Part model, mm, in its own coordinate system. Face numbers are marked on the shaded views. A direction names the side the tool comes from. Coordinates: 2 decimals unless noted, no trailing zeros. Loops run counter-clockwise (first coordinate to the right, second up) from the corner with the lowest first, then second, coordinate; pieces in that order, holes last. Notation, with made-up numbers: (68, 80.5) - (125, 80.5) arc R30 cw to (125, 102.5) - close; hole circle Ø9 at (-23.5, 59.25). An arc over 180 degrees is marked (long way). Use a Markdown table: item, result. Add a question column.
1) Pull direction X, two halves, no side cores. Call the marked faces 3, 4 and 5: +X half, -X half, draft (parallel to the pull), parting line (faces both ways), or undercut.
2) Drop flat-ended pins along their axis: P1, Ø1.5, axis at x = 131, y = 53.5, coming from the +Z side; P2, Ø1.5, axis at x = 109, z = -30, coming from the +Y side. Give the stop position or say it passes through.
3) Probe probe 1 along X at (y, z) = (14.5, -99); probe 2 along Y at (x, z) = (57, -85.5); probe 3 along Z at (x, y) = (65, 60.5). List the from-to ranges inside material, lowest first. Write a range as [from, to].
4) Band-saw the part on B-B (x = 57). Give the cut face in (y, z), plus the area to 3 significant figures.
5) Tool access for the marked faces 1 and 2: list every direction of +Z, -Z, +X, -X, +Y, -Y with a clear straight run to the whole face (end or side of a thin tool).
6) Band-saw the part on C-C (y = 27.5). Give the cut face in (x, z).
7) Band-saw the part on D-D (z = -32.5). Give the cut face in (x, y).
8) Band-saw the part on A-A (z = -102). Give the cut face in (x, y).
from build123d import *

# Parameters (mm, degrees)
SKETCH1_W           = 140
SKETCH1_H           = 120
BOSS_EXTRUDE1_DEPTH = 10
BOSS_EXTRUDE2_DEPTH = 200
SKETCH3_W           = 15
SKETCH3_H           = 3
CUT_EXTRUDE1_DEPTH  = 3
SKETCH4_W           = 15
SKETCH4_H           = 3
CUT_EXTRUDE2_DEPTH  = 3
SKETCH5_W           = 120
SKETCH5_H           = 7.283967232
BOSS_EXTRUDE3_DEPTH = 40
SKETCH6_W           = 120
SKETCH6_H           = 70
BOSS_EXTRUDE4_DEPTH = 79


with BuildPart() as part:
    # Sketch1 → Boss-Extrude1 (new body)
    with BuildSketch(Plane(origin=(0, 0, 0), x_dir=(1, 0, 0), z_dir=(0, 1, 0))):
        with Locations((70, 60)):
            Rectangle(SKETCH1_W, SKETCH1_H)
    extrude(amount=BOSS_EXTRUDE1_DEPTH)

    # Sketch2 → Boss-Extrude2 (add)
    with BuildSketch(Plane(origin=(0, 10, 0), x_dir=(1, 0, 0), z_dir=(0, 1, 0))):
        Polygon((0, 120), (0, 0), (10, 0), (10, 10.536291888), (7, 10.536291888), (7, 13.536291888), (10, 13.536291888), (10, 110), (70, 110), (70, 120), align=None)
        Polygon((130, 10.536291888), (130, 0), (140, 0), (140, 120), (70, 120), (70, 110), (130, 110), (130, 13.536291888), (133, 13.536291888), (133, 10.536291888), align=None)
    extrude(amount=BOSS_EXTRUDE2_DEPTH)

    # Sketch3 → Cut-Extrude1 (cut)
    with BuildSketch(Plane(origin=(10, 0, 0), x_dir=(0, 0, -1), z_dir=(1, 0, 0))):
        with Locations((21.036291888, 177.819120876)):
            Rectangle(SKETCH3_W, SKETCH3_H)
        Polygon((13.536291888, 166.319120876), (13.536291888, 163.319120876), (28.536291888, 163.319120876), (28.536291888, 166.527780645), align=None)
        with Locations((21.036291888, 151.819120876)):
            Rectangle(SKETCH3_W, SKETCH3_H)
        with Locations((21.036291888, 138.819120876)):
            Rectangle(SKETCH3_W, SKETCH3_H)
        with Locations((21.036291888, 125.819120876)):
            Rectangle(SKETCH3_W, SKETCH3_H)
        with Locations((21.036291888, 112.819120876)):
            Rectangle(SKETCH3_W, SKETCH3_H)
        with Locations((21.036291888, 99.819120876)):
            Rectangle(SKETCH3_W, SKETCH3_H)
        with Locations((21.036291888, 86.819120876)):
            Rectangle(SKETCH3_W, SKETCH3_H)
        Polygon((13.536291888, 75), (13.536291888, 72), (28.533994657, 71.737489743), (28.533994657, 75), align=None)
        with Locations((21.036291888, 60.5)):
            Rectangle(SKETCH3_W, SKETCH3_H)
        Polygon((13.536291888, 49), (13.536291888, 46), (28.536291888, 46), (28.536291888, 49), (13.757115753, 49), align=None)
        with Locations((21.036291888, 34.5)):
            Rectangle(SKETCH3_W, SKETCH3_H)
        with Locations((21.036291888, 21.5)):
            Rectangle(SKETCH3_W, SKETCH3_H)
    extrude(amount=-CUT_EXTRUDE1_DEPTH, mode=Mode.SUBTRACT)

    # Sketch4 → Cut-Extrude2 (cut)
    with BuildSketch(Plane.ZY.offset(-130)):
        with Locations((-21.036291888, 21.5)):
            Rectangle(SKETCH4_W, SKETCH4_H)
        with Locations((-21.036291888, 34.5)):
            Rectangle(SKETCH4_W, SKETCH4_H)
        Polygon((-18.143826221, 46), (-13.536291888, 46), (-13.536291888, 49), (-28.536291888, 49), (-28.536291888, 46), align=None)
        with Locations((-21.036291888, 60.5)):
            Rectangle(SKETCH4_W, SKETCH4_H)
        with Locations((-21.036291888, 73.5)):
            Rectangle(SKETCH4_W, SKETCH4_H)
        with Locations((-21.036291888, 86.5)):
            Rectangle(SKETCH4_W, SKETCH4_H)
        with Locations((-21.036291888, 99.5)):
            Rectangle(SKETCH4_W, SKETCH4_H)
        with Locations((-21.036291888, 112.5)):
            Rectangle(SKETCH4_W, SKETCH4_H)
        with Locations((-21.036291888, 125.5)):
            Rectangle(SKETCH4_W, SKETCH4_H)
        with Locations((-21.036291888, 138.5)):
            Rectangle(SKETCH4_W, SKETCH4_H)
        with Locations((-21.036291888, 151.5)):
            Rectangle(SKETCH4_W, SKETCH4_H)
        with Locations((-21.036291888, 164.5)):
            Rectangle(SKETCH4_W, SKETCH4_H)
        with Locations((-21.036291888, 177.5)):
            Rectangle(SKETCH4_W, SKETCH4_H)
    extrude(amount=-CUT_EXTRUDE2_DEPTH, mode=Mode.SUBTRACT)

    # Sketch5 → Boss-Extrude3 (add)
    with BuildSketch(Plane.XY.offset(-110)):
        with Locations((70, 83.641983616)):
            Rectangle(SKETCH5_W, SKETCH5_H)
    extrude(amount=BOSS_EXTRUDE3_DEPTH)

    # Sketch6 → Boss-Extrude4 (add)
    with BuildSketch(Plane.XY):
        with Locations((70, 45)):
            Rectangle(SKETCH6_W, SKETCH6_H)
    extrude(amount=-BOSS_EXTRUDE4_DEPTH)


solid = part.part
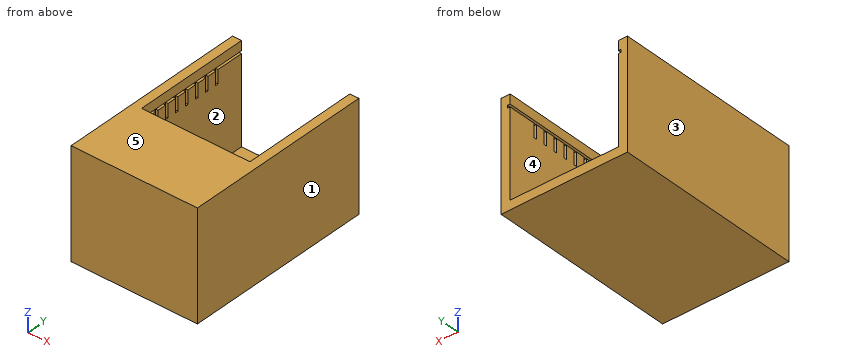
Answer block:
| question | item | result |
|---|---|---|
| 1 | face 3 | -X half |
| 1 | face 4 | undercut |
| 1 | face 5 | draft |
| 2 | P1 | z = 0 |
| 2 | P2 | y = 80 |
| 3 | probe 1 | [0, 10], [130, 140] |
| 3 | probe 2 | [0, 10], [80, 87.28] |
| 3 | probe 3 | [-120, -110], [-79, 0] |
| 4 | outline | (0, -120) - (210, -120) - (210, -110) - (87.28, -110) - (87.28, -70) - (80, -70) - (80, 0) - (0, 0) - close; hole (10, -110) - (80, -110) - (80, -79) - (10, -79) - close |
| 4 | area | 9,020 mm2 |
| 5 | face 1 | +Z, -Z, +X, +Y, -Y |
| 5 | face 2 | +Z, +Y |
| 6 | outline | (0, -120) - (140, -120) - (140, 0) - (0, 0) - close; hole (7, -13.54) - (10, -13.54) - (10, -10.54) - (7, -10.54) - close; hole (10, -110) - (130, -110) - (130, -79) - (10, -79) - close; hole (130, -13.54) - (133, -13.54) - (133, -10.54) - (130, -10.54) - close |
| 7 | outline | (0, 0) - (140, 0) - (140, 210) - (130, 210) - (130, 80) - (10, 80) - (10, 210) - (0, 210) - close |
| 8 | outline | (0, 0) - (140, 0) - (140, 210) - (130, 210) - (130, 87.28) - (10, 87.28) - (10, 210) - (0, 210) - close; hole (10, 10) - (130, 10) - (130, 80) - (10, 80) - close |
